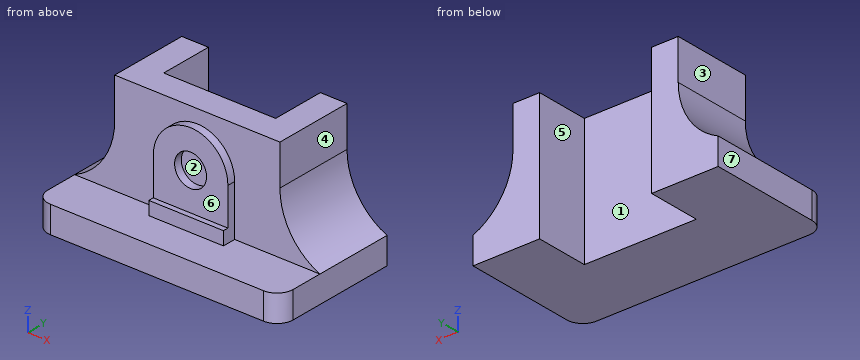
from build123d import *

# Parameters (mm, degrees)
F1_DEPTH = 48
F0_W     = 92
F0_H     = 18
F2_DEPTH = 10
F4_DEPTH = 42.2
F5_R     = 6
F6_DEPTH = 3
F5_W     = 28
F5_H     = 5
F7_DEPTH = 5
F8_R     = 6


with BuildPart() as f1:
    # F0 (on Top) → F1 (new body)
    with BuildSketch(Plane.XY):
        Polygon((-21, 30), (-46, 30), (-46, 0), (46, 0), (46, 30), (21, 30), (21, 10), (-21, 10), align=None)
    extrude(amount=F1_DEPTH)

    # F0 (on Top) → F2 (join)
    with BuildSketch(Plane.XY):
        with Locations((0, -9)):
            Rectangle(F0_W, F0_H)
    extrude(amount=F2_DEPTH)

    # F3 (on Front) → F4 (cut)
    with BuildSketch(Plane.XZ):
        with BuildLine():
            Line((-31, 32.9128784748), (-31, 56.0039258774))
            Line((-31, 56.0039258774), (-46.4185841416, 56.0039258774))
            ThreePointArc((-46.4185841416, 56.0039258774), (-35.208951488, 46.7956844509), (-31, 32.9128784748))
        make_face()
        with BuildLine():
            ThreePointArc((-46.4185841416, 56.0039258774), (-76.791048512, 19.0300724987), (-31, 32.9128784748))
            ThreePointArc((-31, 32.9128784748), (-35.208951488, 46.7956844509), (-46.4185841416, 56.0039258774))
        make_face()
        with BuildLine():
            ThreePointArc((81, 32.9128784748), (69.8828059761, 53.7039269868), (46.4185841416, 56.0039258774))
            ThreePointArc((46.4185841416, 56.0039258774), (35.208951488, 46.7956844509), (31, 32.9128784748))
            ThreePointArc((31, 32.9128784748), (56, 7.9128784748), (81, 32.9128784748))
        make_face()
        with BuildLine():
            ThreePointArc((31, 32.9128784748), (35.208951488, 46.7956844509), (46.4185841416, 56.0039258774))
            Line((46.4185841416, 56.0039258774), (31, 56.0039258774))
            Line((31, 56.0039258774), (31, 32.9128784748))
        make_face()
    extrude(amount=-F4_DEPTH, mode=Mode.SUBTRACT)

    # F5 (on face) → F6 (join)
    with BuildSketch(Plane.XZ):
        with BuildLine():
            Line((14, 15), (14, 29))
            ThreePointArc((14, 29), (0, 43), (-14, 29))
            Line((-14, 29), (-14, 15))
            Line((-14, 15), (14, 15))
        make_face()
        with Locations((0, 29)):
            Circle(F5_R, mode=Mode.SUBTRACT)
    extrude(amount=F6_DEPTH)

    # F5 (on face) → F7 (join)
    with BuildSketch(Plane.XZ):
        with Locations((0, 12.5)):
            Rectangle(F5_W, F5_H)
    extrude(amount=F7_DEPTH)

    # F8
    f8_edges = [f1.edges().sort_by_distance(p)[0] for p in [
        (-46, -18, 5),
        (46, -18, 5),
    ]]
    fillet(f8_edges, radius=F8_R)


solid = f1.part
Model file for the job. Use its own axes, mm. Face numbers are marked on the shaded views. A direction names the side the tool comes from. Coordinates: 2 decimals unless noted, no trailing zeros. Write each loop counter-clockwise with the first axis right and the second up, starting at its lowest first coordinate (ties: lowest second). Pieces come first, ordered by that corner, then holes. Notation, with made-up numbers: (41, -7) -> (87, -7) arc R33 cw to (87, 32) -> close; hole circle Ø7 at (-26.75, 60). An arc over 180 degrees is marked (long way). One line per item, written item: value. Start each with the question number.
1) Slice it at D-D on y = -6. Write the cut outline in (x, z).
2) Probe probe 1 along X at (y, z) = (27.5, 44); probe 2 along Z at (x, y) = (0, -1.95); probe 3 along Y at (x, z) = (4, 42). List the from-to ranges inside material, lowest first.
3) Pull direction X, two halves, no side cores. Call the marked faces 5, 6 and 7: +X half, -X half, draft (parallel to the pull), parting line (faces both ways), or undercut.
4) Slice it at B-B on z = 9. Write the cut outline in (x, y), then the cut area to 3 significant figures.
5) Slice it at A-A on y = 22. Write the cut outline in (x, z), then the cut area to 3 significant figures.
6) Which spindle directions (+Z, -Z, +X, -X, +Y, -Y) get a long thin tool onto all of the face, cutting with end or side? Do the marked faces 1, 2, 3 and 4. Say none if no direction does.
7) Flat gauge pins, fed straight in: pin 1 Ø9 at (x, y) = (13, -6.5) entering from +Z; pin 2 Ø11.5 at (x, z) = (-22.5, 30) entering from -Y; pin 3 Ø2.5 at (y, z) = (-3.5, 22.5) entering from +X. Where does each tip first touch, or does it go through?
8) Slice it at C-C on x = 19. Write the cut outline in (y, z), then the cut area to 3 significant figures.
Answers follow:
1. outline: (-46, 0) -> (46, 0) -> (46, 10) -> (-46, 10) -> close
2. probe 1: -31 to -21, 21 to 31
2. probe 2: 0 to 23, 35 to 43
2. probe 3: -3 to 10
3. face 5: undercut
3. face 6: draft
3. face 7: -X half
4. outline: (-46, -12) arc R6 ccw to (-40, -18) -> (40, -18) arc R6 ccw to (46, -12) -> (46, 30) -> (21, 30) -> (21, 10) -> (-21, 10) -> (-21, 30) -> (-46, 30) -> close
4. area: 3,560 mm2
5. outline: (-46, 0) -> (-21, 0) -> (-21, 48) -> (-31, 48) -> (-31, 32.91) arc R25 cw to (-46, 10) -> close; (21, 0) -> (46, 0) -> (46, 10) arc R25 cw to (31, 32.91) -> (31, 48) -> (21, 48) -> close
5. area: 1,450 mm2
6. face 1: +Z, -Z, +Y
6. face 2: -Y
6. face 3: +Z, -X, +Y, -Y
6. face 4: +Z, +X, +Y, -Y
7. pin 1: z = 38.62
7. pin 2: y = 0
7. pin 3: x = 14
8. outline: (-18, 0) -> (10, 0) -> (10, 48) -> (0, 48) -> (0, 10) -> (-18, 10) -> close
8. area: 660 mm2
